Geometry: final body of the model. Coordinates: model frame, mm. A direction names the side the tool comes from. Round coordinates to 2 decimals unless told otherwise and drop trailing zeros. Loops run counter-clockwise (first coordinate to the right, second up) from the corner with the lowest first, then second, coordinate; pieces in that order, holes last. Notation, with made-up numbers: M 38.25,-21 L 43.25,-21 A18 cw 43.25,0 Z; hole C 49.5,80 d10. An arc over 180 degrees is marked long. Answer as a JSON object with one key per item and string values.
```python
from build123d import *

# Parameters (mm, degrees)
F0_W     = 100
F0_H     = 200
F1_DEPTH = 600
F2_R     = 10
F3_DEPTH = 100


with BuildPart() as f1:
    # F0 (on Front) → F1 (new body)
    with BuildSketch(Plane.XZ):
        with Locations((-50, 100)):
            Rectangle(F0_W, F0_H)
    extrude(amount=F1_DEPTH)

    # F2 (on face) → F3 (cut)
    with BuildSketch(Plane(origin=(0, 0, 0), x_dir=(1, 0, 0), z_dir=(0, 0, -1))):
        with Locations((-50, 430)):
            Circle(F2_R)
        with Locations((-50, 170)):
            Circle(F2_R)
        with Locations((-50, 300)):
            Circle(F2_R)
    extrude(amount=-F3_DEPTH, mode=Mode.SUBTRACT)


solid = f1.part
```
1) Line query: probe 1 along Y at (x, z) = (-50, 38); probe 2 along X at (y, z) = (-300, 20); probe 3 along Y at (x, z) = (-58.5, 62.5). Output: solid intervals per line, ascending.
Geometry results:
{"probe 1": "-600 to -440, -420 to -310, -290 to -180, -160 to 0", "probe 2": "-100 to -60, -40 to 0", "probe 3": "-600 to -435.27, -424.73 to -305.27, -294.73 to -175.27, -164.73 to 0"}
2) Pull-direction query (X, two-part tool) for faces 1 (the face through (-50, -300, 100)), 2 (the face through (-100, -296, 99)), 3 (the face through (-51.302, -439.915, 49.3)), 4 (the face through (-51, -600, 101)); classes: +X half, -X half, draft (parallel to the pull), parting line (faces both ways), or undercut.
Geometry results:
{"face 1": "undercut", "face 2": "-X half", "face 3": "undercut", "face 4": "draft"}
3) Set-up query: faces 5 (the face through (-51, -296, 200)), 6 (the face through (-50, -170, 100)). Return all of +Z, -Z, +X, -X, +Y, -Y with unobstructed straight access to the full face (end or side cutting, diameter ignored); none if empty.
Geometry results:
{"face 5": "+Z, +X, -X, +Y, -Y", "face 6": "-Z"}
4) First-contact query: pin 1 (22 mm diameter, centred on x = -45, y = -431.5, fed in from -Z); pin 2 (10 mm diameter, centred on x = -46.5, y = -303, fed in from -Z). Flat tips, straight axial feed; report the tip coordinate or a pass-through.
Geometry results:
{"pin 1": "z = 0", "pin 2": "z = 100"}
5) Cut plane C-C on y = -170. Return the cut outline in (x, z).
Geometry results:
{"outline": "M -100,0 L -60,0 L -60,100 L -40,100 L -40,0 L 0,0 L 0,200 L -100,200 Z"}
6) Cut plane A-A on z = 93. Return the cut outline in (x, y), and give its area (3 significant figures).
Geometry results:
{"outline": "M -100,-600 L 0,-600 L 0,0 L -100,0 Z; hole C -50,-430 d20; hole C -50,-300 d20; hole C -50,-170 d20", "area": "59,100 mm2"}
7) Cut plane B-B on x = -50. Return the cut outline in (y, z), and give its area (3 significant figures).
Geometry results:
{"outline": "M -600,0 L -440,0 L -440,100 L -420,100 L -420,0 L -310,0 L -310,100 L -290,100 L -290,0 L -180,0 L -180,100 L -160,100 L -160,0 L 0,0 L 0,200 L -600,200 Z", "area": "114,000 mm2"}
